The model under review builds one solid part; all positions refer to its coordinate system, in mm. A direction names the side the tool comes from. Coordinates: 2 decimals unless noted, no trailing zeros. Loops run counter-clockwise (first coordinate to the right, second up) from the corner with the lowest first, then second, coordinate; pieces in that order, holes last. Notation, with made-up numbers: M 27,-3.75 L 57,-3.75 A10 ccw 57,10.25 Z; hole C 88,-29 d8. An arc over 180 degrees is marked long. Use CSV: the item, a comma, the result in double quotes. Start each with the question number.
Autodesk Inventor part; units mm, degrees
ref_plane "YZ Plane" through (0, 0, 0) normal (1, 0, 0) x (0, 1, 0)
ref_plane "XZ Plane" through (0, 0, 0) normal (0, 1, 0) x (-1, 0, 0)
ref_plane "XY Plane" through (0, 0, 0) normal (0, 0, 1) x (1, 0, 0)
sketch "Sketch1" plane through (0, 0, 0) normal (0, 0, 1) x (1, 0, 0)
  line L0 (24.7, 6.5) -> (13, 6.5)
  line L1 (13, 6.5) -> (13, -1.6)
  line L2 (13, -1.6) -> (-13, -1.6)
  line L3 (-13, -1.6) -> (-13, 6.5)
  line L4 (-13, 6.5) -> (-24.7, 6.5)
  line L5 (-24.7, 6.5) -> (-24.7, -6.5)
  line L6 (-24.7, -6.5) -> (24.7, -6.5)
  line L7 (24.7, -6.5) -> (24.7, 6.5)
  line L8 (-24.7, 6.6) -> (24.7, 6.6)
  line L9 (24.7, 6.6) -> (24.7, 9.6)
  line L10 (-24.7, 9.6) -> (24.7, 9.6)
  line L11 (-24.7, 6.6) -> (-24.7, 9.6)
  line L12 (-12.9, -1.5) -> (12.9, -1.5)
  line L13 (12.9, -1.5) -> (12.9, 6.5)
  line L14 (12.9, 6.5) -> (-12.9, 6.5)
  line L15 (-12.9, 6.5) -> (-12.9, -1.5)
  line L16 (11.9, -0.5) -> (-11.9, -0.5)
  line L17 (-11.9, -0.5) -> (-11.9, 5.5)
  line L18 (-11.9, 5.5) -> (11.9, 5.5)
  line L19 (11.9, 5.5) -> (11.9, -0.5)
  point P0 (0, 0)
  dimension "d0" = 0.1
  dimension "d1" = 0.1
  dimension "d2" = 0.1
  dimension "d3" = 0.1
  dimension "d4" = 1
extrude "Extrusion1" add sketch "Sketch1" along normal mid plane 5 contours L15 L14 L13 L12
ref_plane "Work Plane1" through (0, 0, 0.1) normal (0, 0, 1) x (1, 0, 0)
sketch "Sketch2" plane through (0, 0, 0.1) normal (0, 0, 1) x (1, 0, 0)
  line L0 (12.9, -1.5) -> (12.9, 6.5)
  line L1 (12.9, 6.5) -> (-12.9, 6.5)
  line L2 (-12.9, 6.5) -> (-12.9, -1.5)
  line L3 (-12.9, -1.5) -> (12.9, -1.5)
  line L4 (11.9, -0.5) -> (-11.9, -0.5)
  line L5 (-11.9, -0.5) -> (-11.9, 5.5)
  line L6 (-11.9, 5.5) -> (11.9, 5.5)
  line L7 (11.9, 5.5) -> (11.9, -0.5)
  line L8 (-14.9, -3.5) -> (-14.9, 8.5)
  line L9 (-14.9, 8.5) -> (14.9, 8.5)
  line L10 (14.9, 8.5) -> (14.9, -3.5)
  line L11 (14.9, -3.5) -> (-14.9, -3.5)
  point P0 (0, 0)
  dimension "d7" = 2
extrude "Extrusion2" add sketch "Sketch2" along normal up to surface (2.4 mm away) contours L8 L9 L10 L11
sketch "Sketch3" plane through (0, 0, 0) normal (1, 0, 0) x (0, 1, 0)
  line L0 (5.5, -2.5) -> (5.5, 2.5)
  line L1 (5.5, 2.5) -> (12.5, 9.5)
  line L2 (12.5, 9.5) -> (15.5, 9.5)
  line L3 (8.5, 2.5) -> (-3.5, 2.5)
  line L4 (15.5, 9.5) -> (8.5, 2.5)
  line L5 (2.5, 2.5) -> (2.5, -1.8048)
  line L6 (-0.5, 2.5) -> (-7.5, 9.5)
  line L7 (-7.5, 9.5) -> (-10.5, 9.5)
  line L8 (-10.5, 9.5) -> (-3.5, 2.5)
  point P0 (0, 0)
  dimension "d10" = 20
  dimension "d11" = 45
extrude "Extrusion3" add sketch "Sketch3" along normal mid plane 25
sketch "Sketch4" plane through (-12.5, 0, 0) normal (-1, 0, 0) x (0, 0, 1)
  line L0 (9.5, 12.5) -> (9.5, 15.5)
  line L1 (9.5, 15.5) -> (2.5, 8.5)
  line L2 (2.5, 5.5) -> (2.5, 8.5)
  line L3 (2.5, 5.5) -> (9.5, 12.5)
  line L4 (2.5, -3.5) -> (2.5, -0.5)
  line L5 (2.5, -3.5) -> (9.5, -10.5)
  line L6 (9.5, -10.5) -> (9.5, -7.5)
  line L7 (9.5, -7.5) -> (2.5, -0.5)
  line L8 (2.5, -3.5) -> (2.5, 8.5)
  line L9 (9.5, 15.5) -> (9.5, 12.5)
  line L10 (9.5, 12.5) -> (9.5, -7.5)
  point P0 (0, 0)
extrude "Extrusion4" add sketch "Sketch4" along normal up to surface (2.4 mm away)
mirror "Mirror1" about plane through (0, 0, 0) normal (1, 0, 0) of "Extrusion4"
properties part number "solids hopper"
1. For faces 5 (the flat face through (12.9, 2, -1)), 6 (the flat face through (-12.9, 3, -1)), 7 (the flat face through (11.9, 3, 0)), 8 (the flat face through (0, 9, 6)), 9 (the flat face through (0, -3.5, 1)), list the 3-axis set-ups (+Z, -Z, +X, -X, +Y, -Y) from which the entire face can be reached by the end or side of a thin tool; tool diameter is ignored.
2. Add section C-C (z = 4). Write out the cut boundary in (x, y), plus the area to 3 significant figures.
3. Add section A-A (y = 3). Write out the cut boundary in (x, z), plus the area to 3 significant figures.
4. Draft analysis for pull direction Y (two halves, no side actions). For faces 1 (the flat face through (0, -7, 6)), 2 (the flat face through (12.5, 3, 7)), 3 (the flat face through (0, 6.5, -1)), 4 (the flat face through (0, 5.5, 0)), state which applies: released by +Y, released by -Y, zero draft, split by the parting line, or undercut.
5. Insertion check: pin 1 Ø3 at (x, z) = (1, -0.5) entering from -Y; pin 2 Ø3 at (x, y) = (10.5, 12) entering from -Z; pin 3 Ø2 at (y, z) = (2, -2) entering from -X. Each pin has a flat end and moves straight along its axis. Give the tip position at first contact, or say it passes through.
6. Add section D-D (y = 11.75). Write out the cut boundary in (x, z).
7. Add section B-B (x = 8.5). Write out the cut boundary in (y, z).
8. To check wall thickness, follow line 1 along Y through (x, z) = (-7.75, 1.75); line 2 along X through (y, z) = (5.5, 6.25); line 3 along Y through (x, z) = (-8.75, -0.5). State the ranges of each line that lie inside material, in increasing order.
Solved:
1,face 5,"-Z, +X, +Y, -Y"
1,face 6,"-Z, -X, +Y, -Y"
1,face 7,"+Z, -Z"
1,face 8,"+Z"
1,face 9,"-Z, +X, -X, -Y"
2,outline,"M -14.9,-5 L 14.9,-5 L 14.9,10 L -14.9,10 Z; hole M -12.5,-2 L 12.5,-2 L 12.5,7 L -12.5,7 Z"
2,area,"222 mm^2"
3,outline,"M -14.9,0.1 L -12.9,0.1 L -12.9,-2.5 L -11.9,-2.5 L -11.9,2.5 L -12.5,2.5 L -12.5,9.5 L -14.9,9.5 Z; M 11.9,-2.5 L 12.9,-2.5 L 12.9,0.1 L 14.9,0.1 L 14.9,9.5 L 12.5,9.5 L 12.5,2.5 L 11.9,2.5 Z"
3,area,"53.2 mm^2"
4,face 1,"released by -Y"
4,face 2,"undercut"
4,face 3,"released by +Y"
4,face 4,"undercut"
5,pin 1,"stops at y = -3.5"
5,pin 2,"stops at z = 4.5"
5,pin 3,"stops at x = -12.9"
6,outline,"M -14.9,5.75 L 14.9,5.75 L 14.9,9.5 L 12.5,9.5 L 12.5,8.75 L -12.5,8.75 L -12.5,9.5 L -14.9,9.5 Z"
7,outline,"M -10.5,9.5 L -3.5,2.5 L -3.5,0.1 L -1.5,0.1 L -1.5,-2.5 L -0.5,-2.5 L -0.5,2.5 L -7.5,9.5 Z; M 5.5,-2.5 L 6.5,-2.5 L 6.5,0.1 L 8.5,0.1 L 8.5,2.5 L 15.5,9.5 L 12.5,9.5 L 5.5,2.5 Z"
8,line 1,"y = -3.5 to -0.5, 5.5 to 8.5"
8,line 2,"x = -14.9 to -12.5, 12.5 to 14.9"
8,line 3,"y = -1.5 to -0.5, 5.5 to 6.5"
